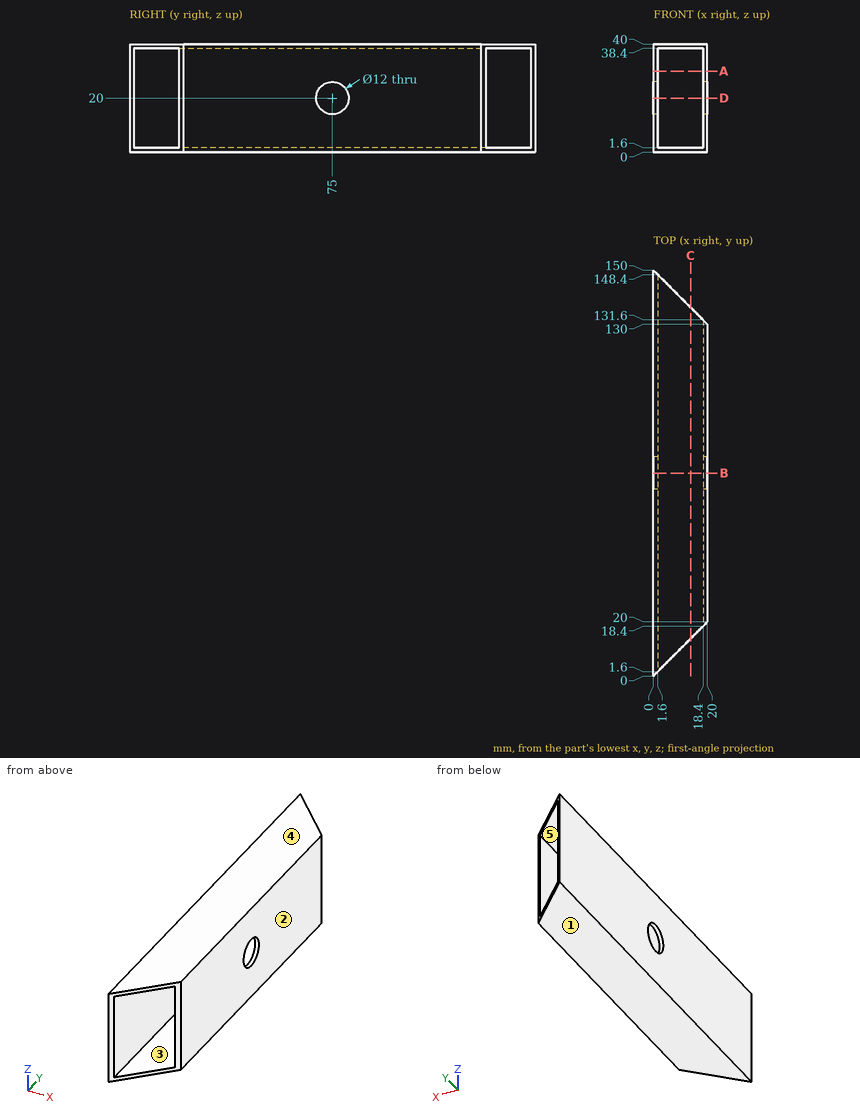
Could you check a few things on this drawing? It's one solid part, dimensions in mm from its lowest x, y, z. A direction names the side the tool comes from. Give positions to 0.01 mm unless a question says otherwise; leave off trailing zeros. Loops run counter-clockwise (first coordinate to the right, second up) from the corner with the lowest first, then second, coordinate; pieces in that order, holes last. Notation, with made-up numbers: M 59,2 L 72,2 A33 ccw 72,41 Z; hole C -24,13 d2. An arc over 180 degrees is marked long. One line per question, with ' | ' between items. Start each with the question number.
Q1. If I drill on line 1 (Z direction, x = 0.6, y = 75); line 2 (X direction, y = 70, z = 37); line 3 (Z direction, x = 9.5, y = 127), over which ranges is the centre line in solid material (lowest first)? Write a range as from..to.
Q2. If we mould it in two halves opening along X, with no side actions, what happens to the marked faces 1, 2 and 3? For each: +X half, -X half, draft (parallel to the pull), parting line (faces both ways), or undercut.
Q3. If we section it at A-A (z = 30): Please give me the cut outline in (x, y), plus the area to 3 significant figures.
Q4. If we section it at B-B (y = 75): Please give me the cut outline in (x, z), plus the area to 3 significant figures.
Q5. If we section it at C-C (x = 13.75): Please give me the cut outline in (y, z), plus the area to 3 significant figures.
Q6. If we section it at D-D (z = 20): Please give me the cut outline in (x, y), plus the area to 3 significant figures.
Q7. For the marked faces 4 and 5, which set-ups out of +Z, -Z, +X, -X, +Y, -Y let a thin tool reach every point of the face, with its end or its side?
Computed:
1) line 1: z = 0..14, 26..40 | line 2: x = 0..1.6, 18.4..20 | line 3: z = 0..1.6, 38.4..40
2) face 1: draft | face 2: +X half | face 3: undercut
3) outline: M 0,0 L 1.6,1.6 L 1.6,148.4 L 0,150 Z; M 18.4,18.4 L 20,20 L 20,130 L 18.4,131.6 Z | area: 416 mm²
4) outline: M 0,0 L 20,0 L 20,14 L 18.4,14 L 18.4,1.6 L 1.6,1.6 L 1.6,14 L 0,14 Z; M 0,26 L 1.6,26 L 1.6,38.4 L 18.4,38.4 L 18.4,26 L 20,26 L 20,40 L 0,40 Z | area: 143 mm²
5) outline: M 13.75,0 L 136.25,0 L 136.25,1.6 L 13.75,1.6 Z; M 13.75,38.4 L 136.25,38.4 L 136.25,40 L 13.75,40 Z | area: 392 mm²
6) outline: M 0,0 L 1.6,1.6 L 1.6,69 L 0,69 Z; M 0,81 L 1.6,81 L 1.6,148.4 L 0,150 Z; M 18.4,18.4 L 20,20 L 20,69 L 18.4,69 Z; M 18.4,81 L 20,81 L 20,130 L 18.4,131.6 Z | area: 378 mm²
7) face 4: +Z, +X, -X, +Y, -Y | face 5: +Y, -Y
